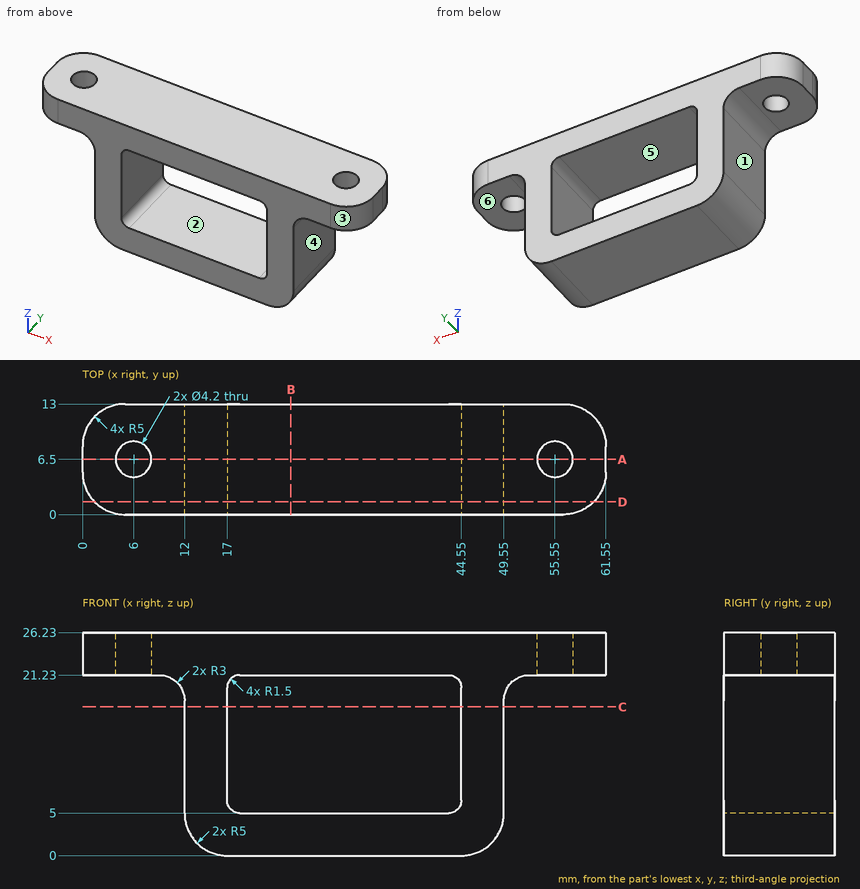
Source: three-view drawing plus pictorial views. Frame: mm from the lowest corner of the part. A direction names the side the tool comes from. Coordinates: 2 decimals unless noted, no trailing zeros. Order: outer loops, then holes, each group sorted by start corner. A loop starts at its lowest first (then second) coordinate and runs counter-clockwise, first axis right, second up. Notation, with made-up numbers: M 71,30.25 L 116,30.25 A11 ccw 116,40.25 Z; hole C 64,31.5 d10. An arc over 180 degrees is marked long. Answer in a Markdown table with one row per item.
(1) Section query D-D, the plane y = 1.5. Output: boundary loops of the cut face in (x, z).
Numbers:
| item | result |
|---|---|
| outline | M 1.43,21.23 L 9,21.23 A3 cw 12,18.23 L 12,5 A5 ccw 17,0 L 44.55,0 A5 ccw 49.55,5 L 49.55,18.23 A3 cw 52.55,21.23 L 60.12,21.23 L 60.12,26.23 L 1.43,26.23 Z; hole M 17,6.5 A1.5 ccw 18.5,5 L 43.05,5 A1.5 ccw 44.55,6.5 L 44.55,19.73 A1.5 ccw 43.05,21.23 L 18.5,21.23 A1.5 ccw 17,19.73 Z |
(2) Material intervals for line 1 (Y direction, x = 55.55, z = 22.9); line 2 (Z direction, x = 37, y = 2); line 3 (Z direction, x = 7.5, y = 1.5), sorted ascending. Write a range as [from, to].
Numbers:
| item | result |
|---|---|
| line 1 | y = [0, 4.4], [8.6, 13] |
| line 2 | z = [0, 5], [21.23, 26.23] |
| line 3 | z = [21.23, 26.23] |
(3) Section query B-B, the plane x = 24.5. Output: boundary loops of the cut face in (y, z), plus the area to 3 significant figures.
Numbers:
| item | result |
|---|---|
| outline | M 0,0 L 13,0 L 13,5 L 0,5 Z; M 0,21.23 L 13,21.23 L 13,26.23 L 0,26.23 Z |
| area | 130 mm^2 |
(4) Contact query for flat-ended pins moving along their axis: pin 1 Ø2.5 at (x, y) = (55.5, 5) entering from -Z; pin 2 Ø1 at (x, y) = (36.5, 6.5) entering from -Z; pin 3 Ø1 at (y, z) = (9, 13) entering from -X; pin 4 Ø4 at (x, y) = (55.55, 6.5) entering from -Z. Output: stop coordinate, or through.
Numbers:
| item | result |
|---|---|
| pin 1 | stops at z = 21.23 |
| pin 2 | stops at z = 0 |
| pin 3 | stops at x = 12 |
| pin 4 | passes through |
(5) Section query A-A, the plane y = 6.5. Output: boundary loops of the cut face in (x, z), plus the area to 3 significant figures.
Numbers:
| item | result |
|---|---|
| outline | M 0,21.23 L 3.9,21.23 L 3.9,26.23 L 0,26.23 Z; M 8.1,21.23 L 9,21.23 A3 cw 12,18.23 L 12,5 A5 ccw 17,0 L 44.55,0 A5 ccw 49.55,5 L 49.55,18.23 A3 cw 52.55,21.23 L 53.45,21.23 L 53.45,26.23 L 8.1,26.23 Z; M 57.65,21.23 L 61.55,21.23 L 61.55,26.23 L 57.65,26.23 Z; hole M 17,6.5 A1.5 ccw 18.5,5 L 43.05,5 A1.5 ccw 44.55,6.5 L 44.55,19.73 A1.5 ccw 43.05,21.23 L 18.5,21.23 A1.5 ccw 17,19.73 Z |
| area | 611 mm^2 |
(6) Section query C-C, the plane z = 17.5. Output: boundary loops of the cut face in (x, y), plus the area to 3 significant figures.
Numbers:
| item | result |
|---|---|
| outline | M 12,0 L 17,0 L 17,13 L 12,13 Z; M 44.55,0 L 49.55,0 L 49.55,13 L 44.55,13 Z |
| area | 130 mm^2 |
(7) Draft query along X for the marked faces 4, 5 and 6. Return one class per face: pulls with the +X half, pulls with the -X half, needs draft (parallel to the pull), parting line crosses it, or undercut.
Numbers:
| item | result |
|---|---|
| face 4 | pulls with the +X half |
| face 5 | undercut |
| face 6 | needs draft |
(8) Access query for the marked faces 1, 2 and 3. Directions: +Z, -Z, +X, -X, +Y, -Y. A direction counts if a zero-diameter tool reaches every point of the face in a straight line with its end or side. Return the directions, or none.
Numbers:
| item | result |
|---|---|
| face 1 | -Z, -X, +Y, -Y |
| face 2 | +Y, -Y |
| face 3 | +Z, -Z, +X, -Y |
